```python
from build123d import *

# Parameters (mm, degrees)
F_10_0_1935_DIAMETER_HOLE1_D       = 4.9149
F_3_16_0_1875_DIAMETER_HOLE1_D     = 4.7625
F_3_16_0_1875_DIAMETER_HOLE1_DEPTH = 6.35
F_3_16_0_1875_DIAMETER_HOLE1_TIP   = 1.430799349
FILLET1_R                          = 2.54
FILLET2_R                          = 1.27
CHAMFER1_SIZE                      = 1.27
F_1_4_0_25_DIAMETER_HOLE2_D        = 6.35
F_1_4_0_25_DIAMETER_HOLE2_DEPTH    = 12.7
F_1_4_0_25_DIAMETER_HOLE2_TIP      = 1.907732465


with BuildPart() as part:
    # Sketch1 → Revolve1 (revolve)
    with BuildSketch(Plane.XY):
        Polygon((-66.802, 50.8), (-66.802, 38.1), (-50.8, 38.1), (-50.8, -50.8), (-41.402, -50.8), (-41.402, 22.225), (-9.525, 22.225), (-9.525, 25.4), (-41.402, 25.4), (-41.402, 47.625), (-50.8, 47.625), (-50.8, 50.8), align=None)
    revolve(axis=Axis((0, 50.8, 0), (0, -1, 0)))

    # #10 (0.1935) Diameter Hole1 (through all)
    with Locations(Plane(origin=(0, 25.4, 0), x_dir=(1, 0, 0), z_dir=(0, 1, 0))):
        with Locations((0, 25.4), (25.4, 0), (0, -25.4), (-25.4, 0)):
            Hole(F_10_0_1935_DIAMETER_HOLE1_D / 2)

    # 3/16 (0.1875) Diameter Hole1
    with Locations(Plane(origin=(0, 47.625, 0), x_dir=(1, 0, 0), z_dir=(0, 1, 0))):
        with Locations((0, 46.355), (46.355, 0), (0, -46.355), (-46.355, 0)):
            Hole(F_3_16_0_1875_DIAMETER_HOLE1_D / 2, depth=F_3_16_0_1875_DIAMETER_HOLE1_DEPTH)
            with Locations((0, 0, -(F_3_16_0_1875_DIAMETER_HOLE1_DEPTH + F_3_16_0_1875_DIAMETER_HOLE1_TIP / 2))):  # 118° drill point
                Cone(0, F_3_16_0_1875_DIAMETER_HOLE1_D / 2, F_3_16_0_1875_DIAMETER_HOLE1_TIP, mode=Mode.SUBTRACT)

    # Fillet1
    fillet1_edges = [part.edges().sort_by_distance(p)[0] for p in [
        (41.402, 22.225, 0),
        (41.402, 25.4, 0),
        (50.8, 38.1, 0),
    ]]
    fillet(fillet1_edges, radius=FILLET1_R)

    # Fillet2
    fillet2_edges = [part.edges().sort_by_distance(p)[0] for p in [
        (50.8, 47.625, 0),
    ]]
    fillet(fillet2_edges, radius=FILLET2_R)

    # Chamfer1
    chamfer1_edges = [part.edges().sort_by_distance(p)[0] for p in [
        (9.525, 22.225, 0),
        (9.525, 25.4, 0),
        (41.402, 47.625, 0),
    ]]
    chamfer(chamfer1_edges, length=CHAMFER1_SIZE)

    # 1/4 (0.25) Diameter Hole2
    with Locations(Plane(origin=(0, 50.8, 0), x_dir=(1, 0, 0), z_dir=(0, 1, 0))):
        with Locations((0, 58.42), (41.309178157, 41.309178157), (58.42, 0), (41.309178157, -41.309178157), (0, -58.42), (-41.309178157, -41.309178157), (-58.42, 0), (-41.309178157, 41.309178157), (0, 0)):
            Hole(F_1_4_0_25_DIAMETER_HOLE2_D / 2, depth=F_1_4_0_25_DIAMETER_HOLE2_DEPTH)
            with Locations((0, 0, -(F_1_4_0_25_DIAMETER_HOLE2_DEPTH + F_1_4_0_25_DIAMETER_HOLE2_TIP / 2))):  # 118° drill point
                Cone(0, F_1_4_0_25_DIAMETER_HOLE2_D / 2, F_1_4_0_25_DIAMETER_HOLE2_TIP, mode=Mode.SUBTRACT)


solid = part.part
```
The model under review builds one solid part; all positions refer to its coordinate system, in mm. A direction names the side the tool comes from. Round coordinates to 2 decimals unless told otherwise and drop trailing zeros. Loops run counter-clockwise (first coordinate to the right, second up) from the corner with the lowest first, then second, coordinate; pieces in that order, holes last. Notation, with made-up numbers: (-2.5, -16) - (21.5, -16) arc R18 cw to (21.5, 8) - close; hole circle Ø5 at (74.5, -11.5). An arc over 180 degrees is marked (long way). Use a Markdown table: item, result. Add a question column.
Q1. Add section B-B (z = 58.42). State the section outline as (x, y) points (3 decimals), plus the area to 3 significant figures.
Q2. Insertion check: pin 1 Ø10 at (y, z) = (37.5, -38.5) entering from +X; pin 2 Ø10 at (x, z) = (-1.5, -17.5) entering from +Y; pin 3 Ø10 at (y, z) = (-9, -47.5) entering from -X; pin 4 Ø4.5 at (x, z) = (25.4, 0) entering from +Y. Each pin has a flat end and moves straight along its axis. Give the tip position at first contact, or say it passes through.
Q3. Machinability: for faces 4 (the face through (25, 38.1, 49)), 5 (the face through (0.69, 44.36, 61.52)), 6 (the face through (33, 37, 25)), which of the approach directions +Z, -Z, +X, -X, +Y, -Y give a long, thin tool a straight path to every point of the face, cutting with its end or side? Answer none if there is none.
Q4. The part is to be moulded in two halves that separate along X. For faces 1 (the face through (27.855, 23.79, -0.108)), 2 (the face through (-25, 50.8, -45)), 3 (the face through (-42.77, 44.36, 44.13)), say which applies: pulls with the +X half, pulls with the -X half, needs draft (parallel to the pull), parting line crosses it, or undercut.
Q5. Add section C-C (y = -26). State the section outline as (x, z) points.
Q6. Add section A-A (x = 58.42). State the section outline as (y, z) points (3 decimals), plus the area to 3 significant figures.
Q7. For probe 1 along Z at (x, y) = (-25.4, 23.4); probe 2 along Z at (x, y) = (-2.5, 39.5); probe 3 along Y at (x, z) = (46, 38), list the stretches that pass through material, from the lowest coordinate up.
Worked answers:
| question | item | result |
|---|---|---|
| 1 | outline | (-32.398, 38.1) - (-3.175, 38.1) - (-3.175, 50.8) - (-32.398, 50.8) - close; (3.175, 38.1) - (32.398, 38.1) - (32.398, 50.8) - (3.175, 50.8) - close |
| 1 | area | 742 mm² |
| 2 | pin 1 | x = 57.77 |
| 2 | pin 2 | y = 25.4 |
| 2 | pin 3 | x = -27.83 |
| 2 | pin 4 | through |
| 3 | face 4 | -Y |
| 3 | face 5 | +Y, -Y |
| 3 | face 6 | +Y |
| 4 | face 1 | undercut |
| 4 | face 2 | needs draft |
| 4 | face 3 | undercut |
| 5 | outline | circle Ø101.6 at (0, 0); hole circle Ø82.8 at (0, 0) |
| 6 | outline | (38.1, -32.398) - (50.8, -32.398) - (50.8, -3.175) - (38.1, -3.175) - close; (38.1, 3.175) - (50.8, 3.175) - (50.8, 32.398) - (38.1, 32.398) - close |
| 6 | area | 742 mm² |
| 7 | probe 1 | -43.99 to -2.46, 2.46 to 43.99 |
| 7 | probe 2 | -66.76 to -60.38, -56.46 to -41.33, 41.33 to 56.46, 60.38 to 66.76 |
| 7 | probe 3 | 38.1 to 50.8 |
